from build123d import *

# Parameters (mm, degrees)
F1_DEPTH = 25
F2_DEPTH = 25


with BuildPart() as f1:
    # F0 (on Front) → F1 (new body)
    with BuildSketch(Plane.XZ):
        with BuildLine():
            ThreePointArc((-14.762832, -18.290401), (-19.327975, 0), (-14.762832, 18.290401))
            ThreePointArc((-14.762832, 18.290401), (-72.201915, 0), (-14.762832, -18.290401))
        make_face()
        with BuildLine():
            ThreePointArc((-14.762832, -18.290401), (-10.429805, -9.597663), (-8.938596, 0))
            ThreePointArc((-8.938596, 0), (-10.429805, 9.597663), (-14.762832, 18.290401))
            ThreePointArc((-14.762832, 18.290401), (-19.327975, 0), (-14.762832, -18.290401))
        make_face()
    extrude(amount=F1_DEPTH)


with BuildPart() as f2:
    # F0 (on Front) → F2 (new body)
    with BuildSketch(Plane.XZ):
        with BuildLine():
            ThreePointArc((-14.762832, 18.290401), (-10.429805, 9.597663), (-8.938596, 0))
            ThreePointArc((-8.938596, 0), (-10.429805, -9.597663), (-14.762832, -18.290401))
            ThreePointArc((-14.762832, -18.290401), (29.020914, -37.764609), (58.518297, 0))
            ThreePointArc((58.518297, 0), (29.020914, 37.764609), (-14.762832, 18.290401))
        make_face()
        with BuildLine():
            ThreePointArc((-14.762832, -18.290401), (-10.429805, -9.597663), (-8.938596, 0))
            ThreePointArc((-8.938596, 0), (-10.429805, 9.597663), (-14.762832, 18.290401))
            ThreePointArc((-14.762832, 18.290401), (-19.327975, 0), (-14.762832, -18.290401))
        make_face()
    extrude(amount=F2_DEPTH)

    # F3: cut F1
    add(f1.part, mode=Mode.SUBTRACT)


solid = f2.part
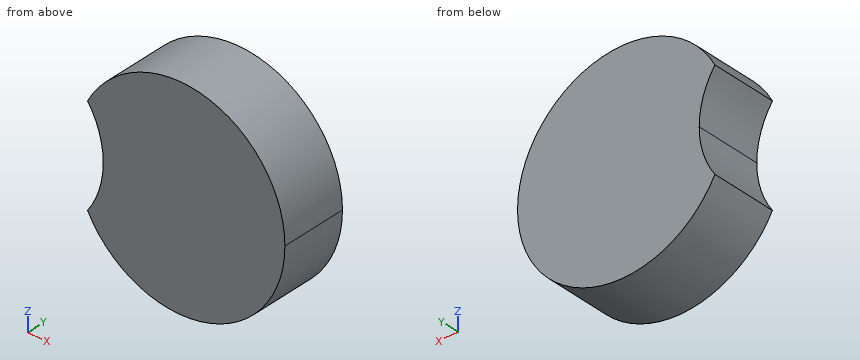
Verification items for the finished model (mm, model axes). Give positions to 0.01 mm unless a question says otherwise; leave off trailing zeros. Order: outer loops, then holes, each group sorted by start corner. A loop starts at its lowest first (then second) coordinate and runs counter-clockwise, first axis right, second up. Notation, with made-up numbers: M -16,-8.75 L 0,-8.75 A15 cw 0,0.25 Z; hole C -18,16.25 d2. An arc over 180 degrees is marked long. Answer as a JSON object with one key per item and string values. Group by question number.
1) Scan lines: line 1 along Z through (x, y) = (19, -17); line 2 along X through (y, z) = (-23.25, -34.5); line 3 along Z through (x, y) = (50.5, -4.25). Record each from-to range of solid material in increasing order. Write a range as [from, to].
2) Depth check by flat-ended pin: pin 1 Ø3 at (x, y) = (16, -4) entering from +Z; pin 2 Ø5 at (x, y) = (-3.5, -9.5) entering from -Z; pin 3 Ø5 at (y, z) = (-20.5, 30.5) entering from -X. Enter the tip coordinate at first touch or a pass-through.
3) Cross-section at A-A (y = -3.5). Enter the section's corners in (x, z), then the cut area to 3 significant figures.
4) Cross-section at B-B (x = 50.5). Enter the section's corners in (y, z).
Result sheet:
{
 "1": {"line 1": "z = [-38.92, 38.92]", "line 2": "x = [1.57, 37.62]", "line 3": "z = [-23.66, 23.66]"},
 "2": {"pin 1": "stops at z = 38.87", "pin 2": "stops at z = -33.03", "pin 3": "stops at x = -7.44"},
 "3": {"outline": "M -14.76,-18.29 A38.92 ccw long -14.76,18.29 A31.63 cw -8.94,0 A31.63 cw Z", "area": "4,500 mm2"},
 "4": {"outline": "M -25,-23.66 L 0,-23.66 L 0,23.66 L -25,23.66 Z"}
}
